The listing builds one solid part. Answer for the finished solid, in the listing's coordinates (mm). Face numbers are marked on the shaded views. A direction names the side the tool comes from. Coordinates: 2 decimals unless noted, no trailing zeros. Order: outer loops, then holes, each group sorted by start corner. A loop starts at its lowest first (then second) coordinate and runs counter-clockwise, first axis right, second up.
from build123d import *

# Parameters (mm, degrees)
F0_W     = 91.42606
F0_H     = 61.178378
F0_W_2   = 76.204642
F0_H_2   = 46.347256
F1_DEPTH = 38.1
F2_W     = 30.83312
F2_H     = 20.100074
F3_DEPTH = 62.738
F4_DEPTH = 41.91
F5_R     = 2.767674
F6_DEPTH = 103.632


with BuildPart() as f1:
    # F0 (on Top) → F1 (new body)
    with BuildSketch(Plane.XY):
        Rectangle(F0_W, F0_H)
        Rectangle(F0_W_2, F0_H_2, mode=Mode.SUBTRACT)
    extrude(amount=F1_DEPTH)

    # F2 (on Front) → F3 (cut)
    with BuildSketch(Plane.XZ):
        with Locations((0.439078, 28.442579)):
            Rectangle(F2_W, F2_H)
    extrude(amount=F3_DEPTH, mode=Mode.SUBTRACT)

    # F2 (on Front) → F4 (cut)
    with BuildSketch(Plane.XZ):
        with Locations((0.439078, 28.442579)):
            Rectangle(F2_W, F2_H)
    extrude(amount=-F4_DEPTH, mode=Mode.SUBTRACT)

    # F5 (on face) → F6 (cut)
    with BuildSketch(Plane.YZ.offset(45.71303)):
        with Locations((0, 26.430823)):
            Circle(F5_R)
    extrude(amount=-F6_DEPTH, mode=Mode.SUBTRACT)


solid = f1.part
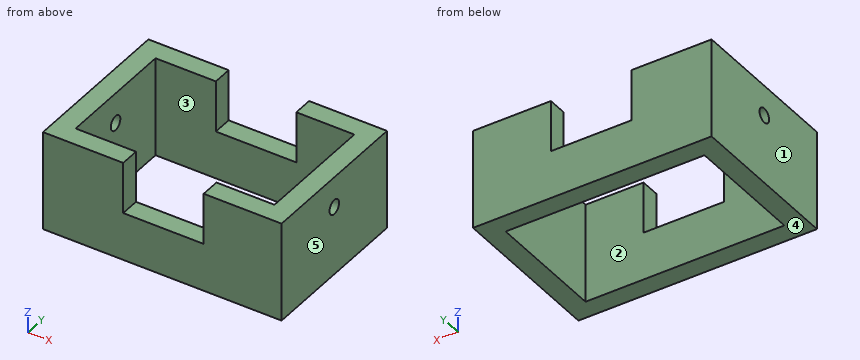
(1) Find section A-A on z = 36. Determine the outline of the cut face in (x, y).
(2) Find section C-C on y = 0. Determine the outline of the cut face in (x, z), then the cut area to 3 significant figures.
(3) Given pin 1 Ø8 at (x, y) = (1.5, -27) entering from +Z; pin 2 Ø8 at (x, y) = (32, -0.5) entering from -Z, each flat-ended and moving along its own axis, determine where each tip first touches the part or whether it passes through.
(4) A tool of negligible diameter and unlimited length cuts with its end or side. For the marked faces 1 and 2, from which of +Z, -Z, +X, -X, +Y, -Y can it reach the whole face along a straight path? Write none if from no direction.
(5) The mould has two halves that part along X. Classify the marked faces 3, 4 and 5: pulls with the +X half, pulls with the -X half, needs draft (parallel to the pull), parting line crosses it, or undercut.
(6) Find section B-B on x = -12.5. Determine the outline of the cut face in (y, z), then the cut area to 3 significant figures.
(7) Find section D-D on z = 11. Determine the outline of the cut face in (x, y).
(8) Find the intervals of material crossed by probe 1 along Z at (x, y) = (-44, 0); probe 2 along X at (y, z) = (-17.5, 5); probe 3 along Y at (x, z) = (15, 17.5), in increasing order.
Resolved:
1. outline: (-45.71, -30.59) - (-14.98, -30.59) - (-14.98, -23.17) - (-38.1, -23.17) - (-38.1, 23.17) - (-14.98, 23.17) - (-14.98, 30.59) - (-45.71, 30.59) - close; (15.86, -30.59) - (45.71, -30.59) - (45.71, 30.59) - (15.86, 30.59) - (15.86, 23.17) - (38.1, 23.17) - (38.1, -23.17) - (15.86, -23.17) - close
2. outline: (-45.71, 0) - (-38.1, 0) - (-38.1, 23.66) - (-45.71, 23.66) - close; (-45.71, 29.2) - (-38.1, 29.2) - (-38.1, 38.1) - (-45.71, 38.1) - close; (38.1, 0) - (45.71, 0) - (45.71, 23.66) - (38.1, 23.66) - close; (38.1, 29.2) - (45.71, 29.2) - (45.71, 38.1) - (38.1, 38.1) - close
2. area: 496 mm2
3. pin 1: stops at z = 18.39
3. pin 2: passes through
4. face 1: +Z, -Z, -X, +Y, -Y
4. face 2: +Z, -Z
5. face 3: undercut
5. face 4: needs draft
5. face 5: pulls with the +X half
6. outline: (-30.59, 0) - (-23.17, 0) - (-23.17, 18.39) - (-30.59, 18.39) - close; (23.17, 0) - (30.59, 0) - (30.59, 18.39) - (23.17, 18.39) - close
6. area: 273 mm2
7. outline: (-45.71, -30.59) - (45.71, -30.59) - (45.71, 30.59) - (-45.71, 30.59) - close; hole (-38.1, -23.17) - (38.1, -23.17) - (38.1, 23.17) - (-38.1, 23.17) - close
8. probe 1: z = 0 to 23.66, 29.2 to 38.1
8. probe 2: x = -45.71 to -38.1, 38.1 to 45.71
8. probe 3: y = -30.59 to -23.17, 23.17 to 30.59
